Input: dimensioned drawing with shaded views. Units: mm. Origin: part minimum x, y, z. Round coordinates to 2 decimals unless told otherwise and drop trailing zeros. Loops run counter-clockwise (first coordinate to the right, second up) from the corner with the lowest first, then second, coordinate; pieces in that order, holes last. Notation, with made-up numbers: M -18.75,83 L 38.25,83 A17 cw 38.25,108 Z; hole C 45.25,-28 d5. An arc over 180 degrees is marked long. One line per item, written item: value.
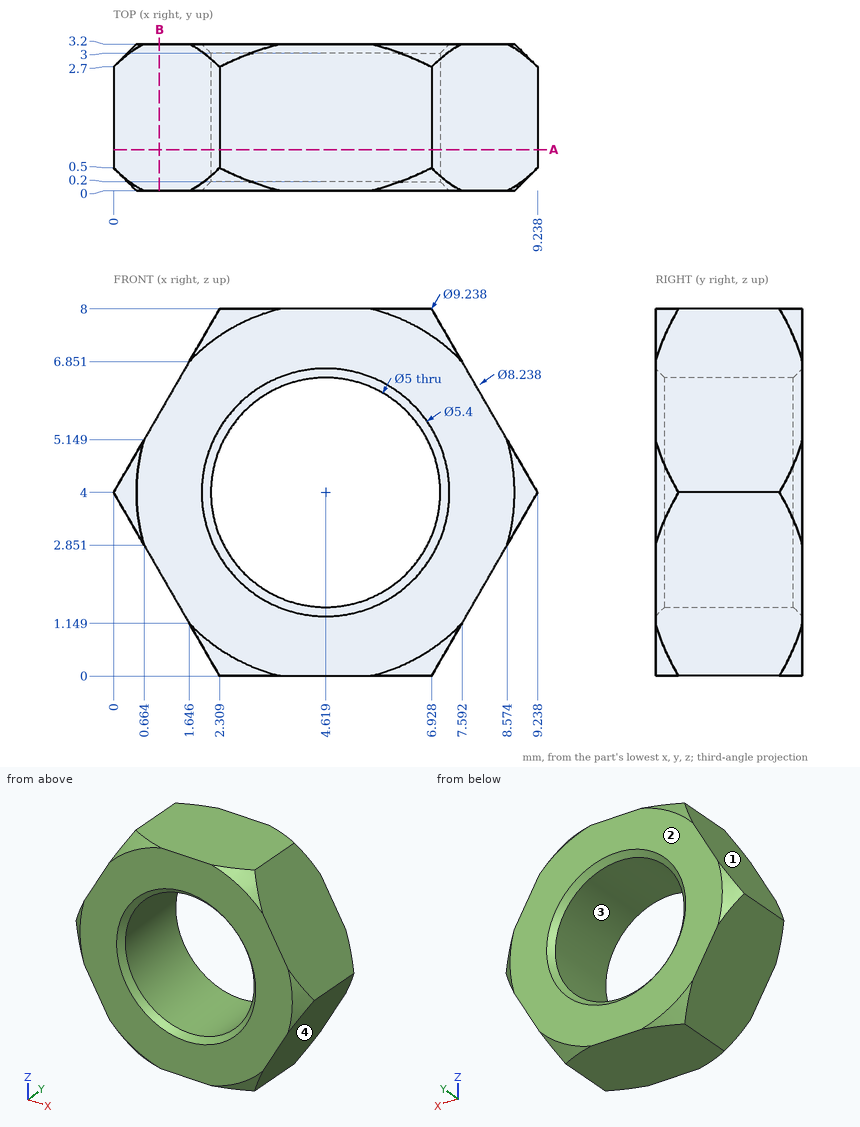
1. Section query B-B (x = 1). Return the cut outline in (y, z).
Report:
outline: M 0,2.27 L 3.2,2.27 L 3.2,5.73 L 0,5.73 Z
2. Ray query, line 1 (Z direction, x = 6, y = 2.9) (1 decimal); line 2 (X direction, y = 2.3, z = 5.5) (1 decimal); line 3 (Z direction, x = 4, y = 2.3). Return the intervals inside material, ascending. Write a range as [from, to].
Report:
line 1: z = [0, 1.9], [6.1, 8]
line 2: x = [0.9, 2.6], [6.6, 8.4]
line 3: z = [0, 1.58], [6.42, 8]
3. Pin query (flat end, axial travel): pin 1 (1 mm diameter, centred on x = 1.5, y = 0.5, fed in from -Z) (1 decimal); pin 2 (1 mm diameter, centred on x = 7.5, y = 1, fed in from -Z) (1 decimal). Return the tip coordinate at first contact, or that it passes through.
Report:
pin 1: stops at z = 0.5
pin 2: stops at z = 0.1
4. Pull-direction query (Z, two-part tool) for the marked faces 1, 2, 3 and 4; classes: released by +Z, released by -Z, zero draft, split by the parting line, or undercut.
Report:
face 1: released by +Z
face 2: zero draft
face 3: undercut
face 4: released by -Z
5. Section query A-A (y = 0.9). Return the cut outline in (x, z).
Report:
outline: M 0,4 L 2.31,0 L 6.93,0 L 9.24,4 L 6.93,8 L 2.31,8 Z; hole C 4.62,4 d5
